from build123d import *

# Parameters (mm, degrees)
F1_DEPTH = 76.2
F2_W     = 17.78
F2_H     = 50.8
F3_DEPTH = 38.1
F5_DEPTH = 63.5
F7_DEPTH = 63.5


with BuildPart() as f1:
    # F0 (on Front) → F1 (new body)
    with BuildSketch(Plane.XZ):
        Polygon((-44.748871, -19.178686), (-44.748871, -44.578686), (44.151129, -44.578686), (44.151129, -19.178686), (18.751129, -19.178686), (18.751129, 44.321314), (44.151129, 44.321314), (44.151129, 69.721314), (-44.748871, 69.721314), (-44.748871, 44.321314), (-19.348871, 44.321314), (-19.348871, -19.178686), align=None)
    extrude(amount=F1_DEPTH)

    # F2 (on face) → F3 (join)
    with BuildSketch(Plane.XY.offset(69.721314)):
        with Locations((-21.511204, -40.512243)):
            Rectangle(F2_W, F2_H)
    extrude(amount=F3_DEPTH)

    # F4 (on face) → F5 (cut)
    with BuildSketch(Plane.YZ.offset(-12.621204)):
        Polygon((-54.192732, 99.692909), (-58.158241, 99.692909), (-58.158241, 82.120264), (-54.192732, 82.120264), (-54.192732, 88.470264), (-50.693755, 88.470264), (-50.693755, 82.120264), (-47.117021, 82.120264), (-47.117021, 99.692909), (-50.693755, 99.692909), (-50.693755, 93.342909), (-54.192732, 93.342909), align=None)
    extrude(amount=-F5_DEPTH, mode=Mode.SUBTRACT)

    # F6 (on face) → F7 (cut)
    with BuildSketch(Plane.YZ.offset(-12.621204)):
        Polygon((-34.177791, 95.228866), (-30.367791, 95.228866), (-30.367791, 99.692909), (-41.473001, 99.692909), (-41.473001, 95.228866), (-37.663001, 95.228866), (-37.663001, 85.972577), (-41.473001, 85.972577), (-41.473001, 82.120264), (-30.367791, 82.120264), (-30.367791, 85.972577), (-34.177791, 85.972577), align=None)
    extrude(amount=-F7_DEPTH, mode=Mode.SUBTRACT)


solid = f1.part
Work out the finished part from the listing and answer in its coordinate system (mm). A direction names the side the tool comes from. Coordinates: 2 decimals unless noted, no trailing zeros. Loops run counter-clockwise (first coordinate to the right, second up) from the corner with the lowest first, then second, coordinate; pieces in that order, holes last. Notation, with made-up numbers: (50.25, -11) -> (61.25, -11) arc R23 ccw to (61.25, 1) -> close; hole circle Ø3 at (25.5, -6.5). An arc over 180 degrees is marked (long way). Answer as CSV lines item,"result".
1) For faces 1 (the face through (-12.621, -41, 89)), 2 (the face through (-21, -41.473, 84)), 3 (the face through (-22, -65.912, 89)), 4 (the face through (32, -38, -19.179)), 5 (the face through (-19.349, -38, 13)), determine the directions among +Z, -Z, +X, -X, +Y, -Y from which every point of the face is accessible in a straight line to the end or side of a thin tool.
A:
face 1,"+Z, +X, +Y, -Y"
face 2,"+X, -X"
face 3,"+Z, +X, -X, -Y"
face 4,"+X, +Y, -Y"
face 5,"-X, +Y, -Y"
2) The part is cut by section A-A (x = 26). Give the vertices of the cut face in (y, z).
A:
outline,"(-76.2, -44.58) -> (0, -44.58) -> (0, -19.18) -> (-76.2, -19.18) -> close; (-76.2, 44.32) -> (0, 44.32) -> (0, 69.72) -> (-76.2, 69.72) -> close"
3) The part is cut by section C-C (x = -7). Give the vertices of the cut face in (y, z), and give its area (3 significant figures).
A:
outline,"(-76.2, -44.58) -> (0, -44.58) -> (0, 69.72) -> (-76.2, 69.72) -> close"
area,"8,710 mm²"
4) Straight lines are drawn through the part: probe 1 along Z at (x, y) = (39.5, -46); probe 2 along Z at (x, y) = (-24.5, -45.5); probe 3 along X at (y, z) = (-63.5, 78). For each, find the intervals that lie inside material, in ascending order.
A:
probe 1,"z = -44.58 to -19.18, 44.32 to 69.72"
probe 2,"z = -44.58 to -19.18, 44.32 to 107.82"
probe 3,"x = -30.4 to -12.62"
5) The part is cut by section D-D (z = 30). Give the vertices of the cut face in (x, y), and give its area (3 significant figures).
A:
outline,"(-19.35, -76.2) -> (18.75, -76.2) -> (18.75, 0) -> (-19.35, 0) -> close"
area,"2,900 mm²"
6) Flat-ended cylindrical pins translate along their axes: pin 1 (6 mm diameter, centred on y = -36.5, z = 27.5, fed in from -X); pin 2 (3 mm diameter, centred on x = -25.5, z = 89.5, fed in from -Y); pin 3 (1.9 mm diameter, centred on x = -20.5, z = 85, fed in from +Y). Find the tip coordinate at first contact, or state that the pin passes through.
A:
pin 1,"stops at x = -19.35"
pin 2,"stops at y = -65.91"
pin 3,"stops at y = -15.11"
7) The part is cut by section B-B (y = -8.5). Give the vertices of the cut face in (x, z), and give its area (3 significant figures).
A:
outline,"(-44.75, -44.58) -> (44.15, -44.58) -> (44.15, -19.18) -> (18.75, -19.18) -> (18.75, 44.32) -> (44.15, 44.32) -> (44.15, 69.72) -> (-44.75, 69.72) -> (-44.75, 44.32) -> (-19.35, 44.32) -> (-19.35, -19.18) -> (-44.75, -19.18) -> close"
area,"6,940 mm²"
8) For a pull along Z with two mould halves and no side action, classify faces 6 (the face through (-1, -38, -44.579)), 7 (the face through (-30.401, -41, 89)), 8 (the face through (-21, -47.117, 91)) as released by +Z, released by -Z, zero draft, split by the parting line, or undercut.
A:
face 6,"released by -Z"
face 7,"zero draft"
face 8,"undercut"
